CAD build for the part. Positions are in the model's coordinates, mm. Give positions to 0.01 mm unless a question says otherwise; leave off trailing zeros. Loops run counter-clockwise (first coordinate to the right, second up) from the corner with the lowest first, then second, coordinate; pieces in that order, holes last.
Autodesk Inventor part; units mm, degrees
ref_plane "YZ Plane" through (0, 0, 0) normal (1, 0, 0) x (0, 1, 0)
ref_plane "XZ Plane" through (0, 0, 0) normal (0, 1, 0) x (-1, 0, 0)
ref_plane "XY Plane" through (0, 0, 0) normal (0, 0, 1) x (1, 0, 0)
sketch "Sketch1" plane through (0, 0, 0) normal (0, 0, 1) x (1, 0, 0)
  line L0 (0, 0) -> (55.4917, 0)
  line L1 (55.4917, 0) -> (55.4917, 55.1277)
  line L2 (55.4917, 55.1277) -> (0, 55.1277)
  line L3 (0, 55.1277) -> (0, 0)
  dimension "d0" = 55.4917
  dimension "d1" = 55.1277
extrude "Extrusion1" add sketch "Sketch1" along normal blind 0.762
sketch "Sketch2" plane through (0, 0, 0.762) normal (0, 0, 1) x (1, 0, 0)
  line L0 (3.0388, 52.072) -> (52.4437, 52.072)
  line L1 (52.4437, 52.072) -> (52.4437, 3.048)
  line L2 (52.4437, 3.048) -> (3.0388, 3.048)
  line L3 (3.0388, 3.048) -> (3.0388, 52.072)
  line L4 (55.4917, 55.1277) -> (0, 55.1277)
  line L5 (55.4917, 0) -> (55.4917, 55.1277)
  line L6 (0, 55.1277) -> (0, 0)
  line L7 (0, 0) -> (55.4917, 0)
  dimension "d4" = 3.0557
  dimension "d5" = 3.048
  dimension "d6" = 3.0388
  dimension "d7" = 3.048
extrude "Extrusion2" add sketch "Sketch2" along normal blind 12.6333
sketch "Sketch3" plane through (0, 0, 0.762) normal (0, 0, 1) x (1, 0, 0)
  line L0 (3.0388, 3.048) -> (3.0388, 52.072)
  line L1 (52.4437, 3.048) -> (52.4437, 52.072)
  line L2 (3.0388, 18.2516) -> (52.4437, 18.2516)
  line L3 (52.4437, 18.2516) -> (52.4437, 16.1969)
  line L4 (52.4437, 16.1969) -> (3.0388, 16.1969)
  line L5 (3.0388, 16.1969) -> (3.0388, 18.2516)
  line L6 (52.4437, 3.048) -> (3.0388, 3.048)
  line L7 (3.0388, 37.0686) -> (52.4437, 37.0686)
  line L8 (52.4437, 37.0686) -> (52.4437, 35.0112)
  line L9 (52.4437, 35.0112) -> (3.0388, 35.0112)
  line L10 (3.0388, 35.0112) -> (3.0388, 37.0686)
  line L11 (3.0388, 52.072) -> (52.4437, 52.072)
  line L12 (3.0388, 3.048) -> (52.4437, 3.048)
  line L13 (27.4802, 3.048) -> (29.5348, 3.048)
  line L14 (29.5348, 3.048) -> (29.5348, 52.072)
  line L15 (29.5348, 52.072) -> (27.4802, 52.072)
  line L16 (27.4802, 52.072) -> (27.4802, 3.048)
  line L17 (5.9731, 52.072) -> (8.0305, 52.072)
  line L18 (8.0305, 52.072) -> (8.0305, 3.048)
  line L19 (8.0305, 3.048) -> (5.9731, 3.048)
  line L20 (5.9731, 3.048) -> (5.9731, 52.072)
  line L21 (47.3023, 52.072) -> (49.3597, 52.072)
  line L22 (49.3597, 52.072) -> (49.3597, 3.048)
  line L23 (49.3597, 3.048) -> (47.3023, 3.048)
  line L24 (47.3023, 3.048) -> (47.3023, 52.072)
  point P0 (0, 0)
  dimension "d10" = 13.1489
  dimension "d11" = 2.0547
  dimension "d12" = 15.0034
  dimension "d13" = 2.0574
  dimension "d14" = 2.0547
  dimension "d15" = 24.4414
  dimension "d16" = 2.0574
  dimension "d17" = 2.9343
  dimension "d18" = 3.084
  dimension "d19" = 2.0574
extrude "Extrusion3" add sketch "Sketch3" along normal blind 12.6333 contours L0 L2 L20 L4 | L20 L4 L18 L6 | L20 L2 L18 L4 | L0 L7 L20 L9 | L20 L9 L18 L2 | L18 L2 L16 L4 | L16 L4 L14 L6 | L20 L7 L18 L9 | L16 L2 L14 L4 | L20 L11 L18 L7 | L18 L7 L16 L9 | L16 L9 L14 L2 | L14 L2 L24 L4 | L24 L4 L22 L6 | L16 L7 L14 L9 | L24 L2 L22 L4 | L16 L11 L14 L7 | L14 L7 L24 L9 | L24 L9 L22 L2 | L22 L2 L1 L4 | L24 L7 L22 L9 | L24 L11 L22 L7 | L22 L7 L1 L9
properties part number "Toy Chassis"
1. Saw through at B-B, the plane y = 41.5. List the corners of the cut face in (x, z), and give its area (3 significant figures).
Responses:
outline: (0, 0) - (55.49, 0) - (55.49, 13.4) - (52.44, 13.4) - (52.44, 0.76) - (49.36, 0.76) - (49.36, 13.4) - (47.3, 13.4) - (47.3, 0.76) - (29.53, 0.76) - (29.53, 13.4) - (27.48, 13.4) - (27.48, 0.76) - (8.03, 0.76) - (8.03, 13.4) - (5.97, 13.4) - (5.97, 0.76) - (3.04, 0.76) - (3.04, 13.4) - (0, 13.4) - close
area: 197 mm2
2. Saw through at A-A, the plane x = 50. List the corners of the cut face in (y, z).
Responses:
outline: (0, 0) - (55.13, 0) - (55.13, 13.4) - (52.07, 13.4) - (52.07, 0.76) - (37.07, 0.76) - (37.07, 13.4) - (35.01, 13.4) - (35.01, 0.76) - (18.25, 0.76) - (18.25, 13.4) - (16.2, 13.4) - (16.2, 0.76) - (3.05, 0.76) - (3.05, 13.4) - (0, 13.4) - close
3. Drop flat-ended pins along their axis: pin 1 (5 mm diameter, centred on x = 5.5, y = 26, fed in from +Z); pin 2 (1.5 mm diameter, centred on x = 42.5, y = 24.5, fed in from +Z). Give the stop position or say it passes through.
Responses:
pin 1: stops at z = 13.4
pin 2: stops at z = 0.76
4. Probe line 1 along Y through (x, z) = (5.5, 3.75); line 2 along X through (y, z) = (51.5, 8.75); line 3 along Z through (x, y) = (21, 39.5). List the from-to ranges inside material, lowest first.
Responses:
line 1: y = 0 to 3.05, 16.2 to 18.25, 35.01 to 37.07, 52.07 to 55.13
line 2: x = 0 to 3.04, 5.97 to 8.03, 27.48 to 29.53, 47.3 to 49.36, 52.44 to 55.49
line 3: z = 0 to 0.76
5. Saw through at C-C, the plane z = 11.5. Count the separate pieces of the cut face and the enclosed holes in it, and give its area (3 significant figures).
Responses:
separate pieces: 1
enclosed holes: 12
area: 1,120 mm2
6. Pull direction Y, two halves, no side cores. Call faces 1 (the face through (28, 32, 13.395)), 2 (the face through (51, 27, 0.762)), 3 (the face through (27, 0, 7)): released by +Y, released by -Y, zero draft, split by the parting line, or undercut.
Responses:
face 1: zero draft
face 2: undercut
face 3: released by -Y
